Design review of the part shown in the three views and the two pictorial views. Dimensions are in mm from the part's minimum x, y and z. Give positions to 0.01 mm unless a question says otherwise; leave off trailing zeros. Write each loop counter-clockwise with the first axis right and the second up, starting at its lowest first coordinate (ties: lowest second). Pieces come first, ordered by that corner, then holes. Notation, with made-up numbers: M 62.25,34 L 118.25,34 A19 cw 118.25,42 Z; hole C 16.5,89.5 d3. An arc over 180 degrees is marked long. Write item = value, one per line.
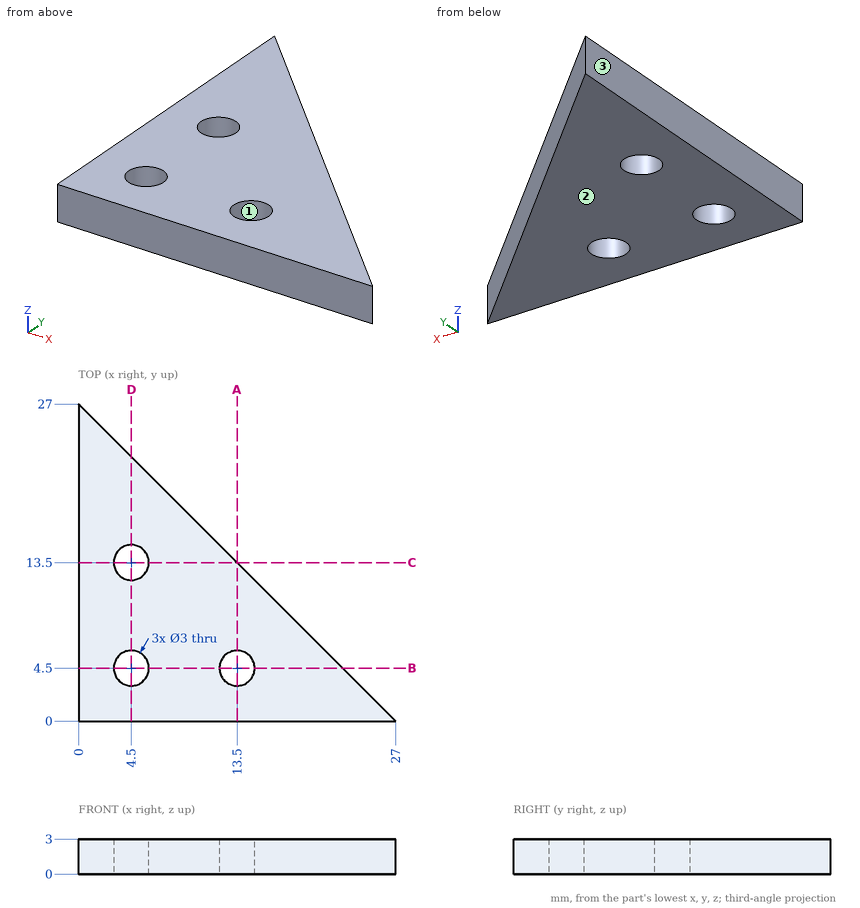
1. We need section A-A, the plane x = 13.5. Write out the cut boundary in (y, z).
Responses:
outline = M 0,0 L 3,0 L 3,3 L 0,3 Z; M 6,0 L 13.5,0 L 13.5,3 L 6,3 Z
2. We need section B-B, the plane y = 4.5. Write out the cut boundary in (x, z), then the cut area to 3 significant figures.
Responses:
outline = M 0,0 L 3,0 L 3,3 L 0,3 Z; M 6,0 L 12,0 L 12,3 L 6,3 Z; M 15,0 L 22.5,0 L 22.5,3 L 15,3 Z
area = 49.5 mm2
3. For line 1 along Y through (x, z) = (4.5, 1.65); line 2 along Y through (x, z) = (5.5, 0.2); line 3 along X through (y, z) = (4.75, 1.45), list the stretches that pass through material, from the lowest coordinate up. Write a range as from..to.
Responses:
line_1 = 0..3, 6..12, 15..22.5
line_2 = 0..3.38, 5.62..12.38, 14.62..21.5
line_3 = 0..3.02, 5.98..12.02, 14.98..22.25
4. The part is to be moulded in two halves that separate along X. For the marked faces 1, 2 and 3, say which applies: +X half, -X half, draft (parallel to the pull), parting line (faces both ways), or undercut.
Responses:
face_1 = undercut
face_2 = draft
face_3 = -X half
5. Insertion check: P1, Ø1.5, axis at y = 14.5, z = 0.5, coming from the +X side; P2, Ø1.5, axis at y = 16, z = 0.5, coming from the +X side; P3, Ø1, axis at x = 7, z = 0.5, coming from the +Y side. Each pin has a flat end and moves straight along its axis. Give the tip position at first contact, or say it passes through.
Responses:
P1 = 13.25
P2 = 11.75
P3 = 20.5
